```python
from build123d import *

# Parameters (mm, degrees)
F2_DEPTH = 2.5
F3_DEPTH = 1
F5_DEPTH = 1
F7_DEPTH = 4.5


with BuildPart() as f2:
    # F1 (on Top) → F2 (new body)
    with BuildSketch(Plane.XY):
        with BuildLine():
            ThreePointArc((9.411918, 9.106117), (9.209323, 9.504574), (8.853362, 9.774952))
            Line((8.853362, 9.774952), (-16.588413, 21.264786))
            ThreePointArc((-16.588413, 21.264786), (-17.542408, 21.193531), (-18, 20.353416))
            Line((-18, 20.353416), (-18, -22))
            ThreePointArc((-18, -22), (-17.707107, -22.707107), (-17, -23))
            Line((-17, -23), (16.157671, -23))
            ThreePointArc((16.157671, -23), (16.945876, -22.615412), (17.127813, -21.757464))
            Line((17.127813, -21.757464), (9.411918, 9.106117))
        make_face()
    extrude(amount=F2_DEPTH)

    # F0 (on Top) → F3 (join)
    with BuildSketch(Plane.XY):
        with BuildLine():
            Line((-18, -25), (17.438447, -25))
            ThreePointArc((17.438447, -25), (19.014858, -24.230824), (19.378732, -22.514929))
            Line((19.378732, -22.514929), (11.234802, 10.060792))
            ThreePointArc((11.234802, 10.060792), (10.829612, 10.857706), (10.11769, 11.398462))
            Line((10.11769, 11.398462), (-17.176827, 23.725018))
            ThreePointArc((-17.176827, 23.725018), (-19.084816, 23.582507), (-20, 21.902277))
            Line((-20, 21.902277), (-20, -23))
            ThreePointArc((-20, -23), (-19.414214, -24.414214), (-18, -25))
        make_face()
    extrude(amount=-F3_DEPTH)

    # F4 (on face) → F5 (join)
    with BuildSketch(Plane.XY.offset(2.5)):
        with BuildLine():
            Line((19.378732, -22.514929), (11.234802, 10.060792))
            ThreePointArc((11.234802, 10.060792), (10.829612, 10.857706), (10.11769, 11.398462))
            Line((10.11769, 11.398462), (-17.176827, 23.725018))
            ThreePointArc((-17.176827, 23.725018), (-19.084816, 23.582507), (-20, 21.902277))
            Line((-20, 21.902277), (-20, -23))
            ThreePointArc((-20, -23), (-19.414214, -24.414214), (-18, -25))
            Line((-18, -25), (17.438447, -25))
            ThreePointArc((17.438447, -25), (19.014858, -24.230824), (19.378732, -22.514929))
        make_face()
        with BuildLine():
            ThreePointArc((8.853362, 9.774952), (9.209323, 9.504574), (9.411918, 9.106117))
            Line((9.411918, 9.106117), (17.127813, -21.757464))
            ThreePointArc((17.127813, -21.757464), (16.945876, -22.615412), (16.157671, -23))
            Line((16.157671, -23), (-17, -23))
            ThreePointArc((-17, -23), (-17.707107, -22.707107), (-18, -22))
            Line((-18, -22), (-18, 20.353416))
            ThreePointArc((-18, 20.353416), (-17.542408, 21.193531), (-16.588413, 21.264786))
            Line((-16.588413, 21.264786), (8.853362, 9.774952))
        make_face(mode=Mode.SUBTRACT)
        with BuildLine():
            Line((17.127813, -21.757464), (9.411918, 9.106117))
            ThreePointArc((9.411918, 9.106117), (9.209323, 9.504574), (8.853362, 9.774952))
            Line((8.853362, 9.774952), (-16.588413, 21.264786))
            ThreePointArc((-16.588413, 21.264786), (-17.542408, 21.193531), (-18, 20.353416))
            Line((-18, 20.353416), (-18, -22))
            ThreePointArc((-18, -22), (-17.707107, -22.707107), (-17, -23))
            Line((-17, -23), (16.157671, -23))
            ThreePointArc((16.157671, -23), (16.945876, -22.615412), (17.127813, -21.757464))
        make_face()
    extrude(amount=F5_DEPTH)

    # F6 (on face) → F7 (cut)
    with BuildSketch(Plane.XY.offset(3.5)):
        with BuildLine():
            ThreePointArc((13.596118, -21), (14.384323, -20.615412), (14.56626, -19.757464))
            Line((14.56626, -19.757464), (7.706434, 7.681839))
            ThreePointArc((7.706434, 7.681839), (7.503839, 8.080295), (7.147879, 8.350674))
            Line((7.147879, 8.350674), (-14.588414, 18.167064))
            ThreePointArc((-14.588414, 18.167064), (-15.542409, 18.095808), (-16.000001, 17.255693))
            Line((-16.000001, 17.255693), (-16.000001, -20))
            ThreePointArc((-16.000001, -20), (-15.707107, -20.707107), (-15.000001, -21))
            Line((-15.000001, -21), (13.596118, -21))
        make_face()
    extrude(amount=-F7_DEPTH, mode=Mode.SUBTRACT)


solid = f2.part
```
The listing builds one solid part. Answer for the finished solid, in the listing's coordinates (mm). A direction names the side the tool comes from. Round coordinates to 2 decimals unless told otherwise and drop trailing zeros. Order: outer loops, then holes, each group sorted by start corner. A loop starts at its lowest first (then second) coordinate and runs counter-clockwise, first axis right, second up. Notation, with made-up numbers: (36, 48) -> (68, 48) arc R32 cw to (68, 77) -> close; hole circle Ø3 at (-18, 6). An arc over 180 degrees is marked (long way). Answer as CSV lines item,"result".
Q1. A cutting plane is placed at B-B on y = 1.5. Determine the outline of the cut face in (x, z) (3 decimals), plus the area to 3 significant figures.
Computed values:
outline,"(-20, -1) -> (-16, -1) -> (-16, 3.5) -> (-20, 3.5) -> (-20, 2.5) -> (-18, 2.5) -> (-18, 0) -> (-20, 0) -> close; (9.252, -1) -> (13.375, -1) -> (13.375, 0) -> (11.313, 0) -> (11.313, 2.5) -> (13.375, 2.5) -> (13.375, 3.5) -> (9.252, 3.5) -> close"
area,"26.4 mm^2"
Q2. Which of the six approach directions +Z, -Z, +X, -X, +Y, -Y give full straight-line access (tool end or side, diameter ignored) to faces 1 (the flat face through (-3.69, 15.44, 1.23)), 2 (the cylindrical face through (-15.715, -20.699, 1.281)), 3 (the flat face through (-20, 0, 3)), 4 (the flat face through (-1, -23, 1))?
Computed values:
face 1,"+X, +Y"
face 2,"+Z, -Z"
face 3,"+Z, -Z, -X, +Y, -Y"
face 4,"+X, -X, -Y"
Q3. A cutting plane is placed at C-C on x = -3. Determine the outline of the cut face in (y, z), plus the area to 3 significant figures.
Computed values:
outline,"(-25, -1) -> (-21, -1) -> (-21, 3.5) -> (-25, 3.5) -> (-25, 2.5) -> (-23, 2.5) -> (-23, 0) -> (-25, 0) -> close; (12.93, -1) -> (17.32, -1) -> (17.32, 0) -> (15.13, 0) -> (15.13, 2.5) -> (17.32, 2.5) -> (17.32, 3.5) -> (12.93, 3.5) -> close"
area,"27.3 mm^2"
Q4. Consider line 1 (X direction, y = -22, z = 0.1); line 2 (X direction, y = -13, z = 0.85); line 3 (X direction, y = 9, z = 1.2). Determine where each line is inside the solid, lowest interval first. Write a range as from..to.
Computed values:
line 1,"x = -18..17.16"
line 2,"x = -18..-16, 12.88..14.94"
line 3,"x = -18..-16, 5.71..9.44"
Q5. For a pull along Z with two mould halves and no side action, classify faces 5 (the cylindrical face through (16.938, -22.625, 1.232)), 6 (the flat face through (-16.4, -4.1, 3.5)), 7 (the flat face through (-1, -21, 1)) as +Z half, -Z half, draft (parallel to the pull), parting line (faces both ways), or undercut.
Computed values:
face 5,"undercut"
face 6,"+Z half"
face 7,"draft"
Q6. Given pin 1 (1.5 mm diameter, centred on x = 3.5, y = -20, fed in from -Z); pin 2 (1.2 mm diameter, centred on y = 2.5, z = 1, fed in from -X); pin 3 (1.3 mm diameter, centred on x = -7, z = 2, fed in from +Y), each flat-ended and moving along its own axis, determine where each tip first touches the part or whether it passes through.
Computed values:
pin 1,"passes through"
pin 2,"stops at x = -18"
pin 3,"stops at y = 19.32"
Q7. A cutting plane is placed at A-A on z = 1.65. Determine the outline of the cut face in (x, y).
Computed values:
outline,"(-18, -22) arc R1 ccw to (-17, -23) -> (16.16, -23) arc R1 ccw to (17.13, -21.76) -> (9.41, 9.11) arc R1 ccw to (8.85, 9.77) -> (-16.59, 21.26) arc R1 ccw to (-18, 20.35) -> close; hole (-16, -20) arc R1 ccw to (-15, -21) -> (13.6, -21) arc R1 ccw to (14.57, -19.76) -> (7.71, 7.68) arc R1 ccw to (7.15, 8.35) -> (-14.59, 18.17) arc R1 ccw to (-16, 17.26) -> close"
